Can you work these out from the model? Positions are in its coordinate system, mm. Face numbers are marked on the shaded views. A direction names the side the tool comes from. Coordinates: 2 decimals unless noted, no trailing zeros. Loops run counter-clockwise (first coordinate to the right, second up) from the corner with the lowest first, then second, coordinate; pieces in that order, holes last.
```python
from build123d import *

# Parameters (mm, degrees)
F1_DEPTH = 140
F2_T     = -2
F3_R     = 3


with BuildPart() as f1:
    # F0 (on Front) → F1 (new body)
    with BuildSketch(Plane.XZ):
        Polygon((0, -93.947366), (-140, 46.052634), (-140, -93.947366), align=None)
    extrude(amount=F1_DEPTH)

    # F2
    f2_openings = [f1.faces().sort_by_distance(p)[0] for p in [
        (-70, -70, -23.947366),
    ]]
    offset(amount=F2_T, openings=f2_openings)

    # F3
    f3_edges = [f1.edges().sort_by_distance(p)[0] for p in [
        (-140, -70, -93.947366),
        (-140, 0, -23.947366),
        (-70, 0, -93.947366),
        (-70, -140, -93.947366),
        (-140, -140, -23.947366),
    ]]
    fillet(f3_edges, radius=F3_R)


solid = f1.part
```
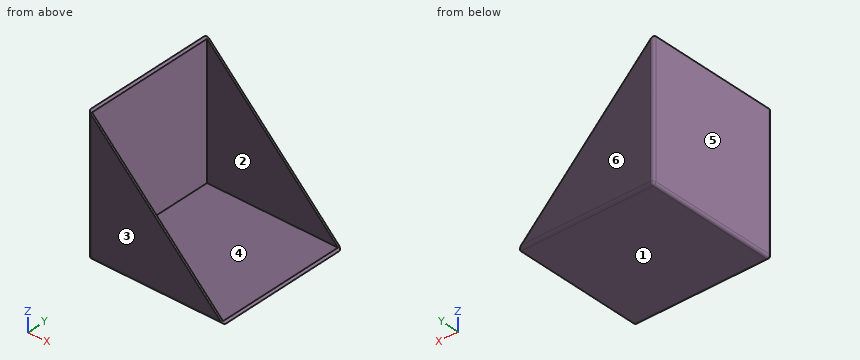
(1) I want a section at A-A on y = -60.5. Write out the boundary of the cut face in (x, z), then the cut area to 3 significant figures.
Check values:
outline: (-140, -90.95) arc R3 ccw to (-137, -93.95) - (0, -93.95) - (-2, -91.95) - (-138, -91.95) - (-138, 44.05) - (-140, 46.05) - close
area: 550 mm2
(2) I'm going to push flat-ended pins straight in: pin 1 (1.5 mm diameter, centred on x = -19, y = -47, fed in from +Z); pin 2 (4 mm diameter, centred on x = -116, z = 25.5, fed in from -Y); pin 3 (8 mm diameter, centred on y = -70.5, z = -69.5, fed in from +X). Where does each tip first touch, or does it pass through?
Check values:
pin 1: stops at z = -91.95
pin 2: passes through
pin 3: stops at x = -138
(3) Which directions (+Z, -Z, +X, -X, +Y, -Y) give clear straight access to the entire face, cutting with the end or side of a thin tool? Please do the marked faces 1 and 2.
Check values:
face 1: -Z, +X, -X, +Y, -Y
face 2: +Z, +X
(4) I want a section at C-C on z = -3. Write out the boundary of the cut face in (x, y), then the cut area to 3 significant figures.
Check values:
outline: (-140, -137) arc R3 ccw to (-137, -140) - (-90.95, -140) - (-90.95, -138) - (-138, -138) - (-138, -2) - (-90.95, -2) - (-90.95, 0) - (-137, 0) arc R3 ccw to (-140, -3) - close
area: 464 mm2
(5) If I drill on probe 1 along Y at (x, z) = (-102, -31.5); probe 2 along Z at (x, y) = (-57.5, -119); probe 3 along X at (y, z) = (-106, 16.5), over which ranges is the centre line in solid material (lowest first)?
Check values:
probe 1: y = -140 to -138, -2 to 0
probe 2: z = -93.95 to -91.95
probe 3: x = -140 to -138
(6) I want a section at B-B on x = -81. Write out the boundary of the cut face in (y, z), then the cut area to 3 significant figures.
Check values:
outline: (-140, -90.95) arc R3 ccw to (-137, -93.95) - (-3, -93.95) arc R3 ccw to (0, -90.95) - (0, -12.95) - (-2, -12.95) - (-2, -91.95) - (-138, -91.95) - (-138, -12.95) - (-140, -12.95) - close
area: 592 mm2
(7) If we mould it in two halves opening along Y, with no side actions, what happens to the marked faces 3, 4, 5 and 6? For each: released by +Y, released by -Y, zero draft, split by the parting line, or undercut.
Check values:
face 3: released by -Y
face 4: undercut
face 5: zero draft
face 6: released by +Y
